Source: CAD feature listing. Evaluate the final solid. Frame: model axes, mm. Give positions to 0.01 mm unless a question says otherwise; leave off trailing zeros. Order: outer loops, then holes, each group sorted by start corner. A loop starts at its lowest first (then second) coordinate and runs counter-clockwise, first axis right, second up. Notation, with made-up numbers: (49.25, -7.5) -> (108.25, -7.5) arc R32 ccw to (108.25, 29.5) -> close; hole circle Ø3 at (81, -11.5). An arc over 180 degrees is marked (long way). Use CSV: the item, a comma, the result in double quotes.
```python
from build123d import *

# Parameters (mm, degrees)
F0_R     = 6.35
F0_R_2   = 3.175
F1_DEPTH = 4.7752


with BuildPart() as f1:
    # F0 (on Front) → F1 (new body)
    with BuildSketch(Plane.XZ):
        with BuildLine():
            Line((47.625, 90.4875), (-47.625, 90.4875))
            Line((-47.625, 90.4875), (-47.625, -42.8625))
            ThreePointArc((-47.625, -42.8625), (-33.67596, -76.53846), (0, -90.4875))
            ThreePointArc((0, -90.4875), (33.67596, -76.53846), (47.625, -42.8625))
            Line((47.625, -42.8625), (47.625, 90.4875))
        make_face()
        with Locations((0, -49.2125)):
            Circle(F0_R, mode=Mode.SUBTRACT)
        with Locations((-34.925, 65.0875)):
            Circle(F0_R_2, mode=Mode.SUBTRACT)
        with Locations((0, 65.0875)):
            Circle(F0_R_2, mode=Mode.SUBTRACT)
        with Locations((34.925, 65.0875)):
            Circle(F0_R_2, mode=Mode.SUBTRACT)
    extrude(amount=F1_DEPTH)


solid = f1.part
```
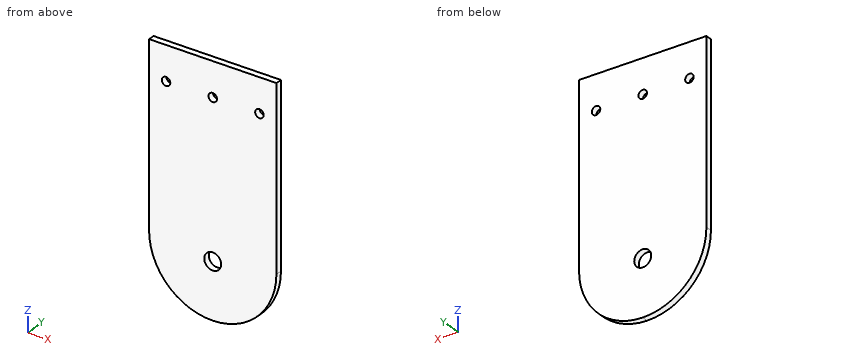
1. Pin query (flat end, axial travel): P1, Ø4, axis at x = -34.92, z = 65.09, coming from the -Y side. Return the tip coordinate at first contact, or that it passes through.
Answer below:
P1,"passes through"
2. Ray query, line 1 along Z through (x, y) = (34.5, -2.85); line 2 along Z through (x, y) = (36, -4); line 3 along Z through (x, y) = (-13.5, -2.85). Return the intervals inside material, ascending.
Answer below:
line 1,"z = -75.69 to 61.94, 68.23 to 90.49"
line 2,"z = -74.04 to 62.1, 68.07 to 90.49"
line 3,"z = -88.53 to 90.49"
3. Section query B-B on z = -53. Return loops of the section in (x, y).
Answer below:
outline,"(-46.53, -4.78) -> (-5.1, -4.78) -> (-5.1, 0) -> (-46.53, 0) -> close; (5.1, -4.78) -> (46.53, -4.78) -> (46.53, 0) -> (5.1, 0) -> close"
4. Section query A-A on y = -2.7. Count the separate pieces of the cut face and the enclosed holes in it, plus the area to 3 significant figures.
Answer below:
separate pieces,"1"
enclosed holes,"4"
area,"16,000 mm²"
5. Section query D-D on x = -23.5. Return loops of the section in (y, z).
Answer below:
outline,"(-4.78, -84.29) -> (0, -84.29) -> (0, 90.49) -> (-4.78, 90.49) -> close"
6. Section query C-C on x = 21.5. Return loops of the section in (y, z).
Answer below:
outline,"(-4.78, -85.36) -> (0, -85.36) -> (0, 90.49) -> (-4.78, 90.49) -> close"
